Build history of the part. All positions in model axes, mm. A direction names the side the tool comes from. Round coordinates to 2 decimals unless told otherwise and drop trailing zeros. Loops run counter-clockwise (first coordinate to the right, second up) from the corner with the lowest first, then second, coordinate; pieces in that order, holes last.
from build123d import *

# Parameters (mm, degrees)
SKETCH1_W           = 127
SKETCH1_H           = 112.8776
BOSS_EXTRUDE1_DEPTH = 1.778
SKETCH2_R           = 1.27
CUT_EXTRUDE1_DEPTH  = 1.778
BOSS_EXTRUDE2_DEPTH = 9.525
SKETCH4_R           = 1.524
CUT_EXTRUDE2_DEPTH  = 1.0922
LPATTERN1_COUNT     = 2
LPATTERN1_PITCH     = 13.589
BOSS_EXTRUDE3_DEPTH = 9.652
SKETCH6_R           = 1.524
CUT_EXTRUDE3_DEPTH  = 1.016
FILLET1_R           = 1.524
FILLET2_R           = 0.508
LPATTERN2_COUNT     = 2
LPATTERN2_PITCH     = 13.0048
SKETCH7_R           = 1.524
CUT_EXTRUDE4_DEPTH  = 1.016
FILLET3_R           = 0.508
FILLET4_R           = 1.524
SKETCH8_R           = 4.445
BOSS_EXTRUDE4_DEPTH = 8.89


with BuildPart() as part:
    # Sketch1 → Boss-Extrude1 (new body)
    with BuildSketch(Plane(origin=(0, 0, 0), x_dir=(1, 0, 0), z_dir=(0, 1, 0))):
        Rectangle(SKETCH1_W, SKETCH1_H)
    extrude(amount=BOSS_EXTRUDE1_DEPTH)

    # Sketch2 → Cut-Extrude1 (cut)
    with BuildSketch(Plane(origin=(0, 1.778, 0), x_dir=(1, 0, 0), z_dir=(0, 1, 0))):
        with Locations((58.42, 52.1208)):
            Circle(SKETCH2_R)
        with Locations((58.42, -52.1208)):
            Circle(SKETCH2_R)
    extrude(amount=-CUT_EXTRUDE1_DEPTH, mode=Mode.SUBTRACT)

    # Sketch3 → Boss-Extrude2 (add)
    with BuildSketch(Plane(origin=(63.5, 0, 0), x_dir=(0, 0, -1), z_dir=(1, 0, 0))):
        with BuildLine():
            Line((-46.8884, 1.778), (-46.8884, 6.7818))
            ThreePointArc((-46.8884, 6.7818), (-46.739610245, 7.141010245), (-46.3804, 7.2898))
            Line((-46.3804, 7.2898), (-38.4556, 7.2898))
            ThreePointArc((-38.4556, 7.2898), (-38.096389755, 7.141010245), (-37.9476, 6.7818))
            Line((-37.9476, 6.7818), (-37.9476, 1.778))
            Line((-37.9476, 1.778), (-36.8554, 1.778))
            Line((-36.8554, 1.778), (-36.8554, 6.7818))
            ThreePointArc((-36.8554, 6.7818), (-37.324087729, 7.913312271), (-38.4556, 8.382))
            Line((-38.4556, 8.382), (-46.3804, 8.382))
            ThreePointArc((-46.3804, 8.382), (-47.511912271, 7.913312271), (-47.9806, 6.7818))
            Line((-47.9806, 6.7818), (-47.9806, 1.778))
            Line((-47.9806, 1.778), (-46.8884, 1.778))
        make_face()
    boss_extrude2 = extrude(amount=-BOSS_EXTRUDE2_DEPTH)

    # Sketch4 → Cut-Extrude2 (cut)
    with BuildSketch(Plane(origin=(0, 8.382, 0), x_dir=(1, 0, 0), z_dir=(0, 1, 0))):
        with Locations((58.7375, -42.418)):
            Circle(SKETCH4_R)
    cut_extrude2 = extrude(amount=-CUT_EXTRUDE2_DEPTH, mode=Mode.SUBTRACT)

    # LPattern1: Boss-Extrude2, Cut-Extrude2 ×2
    with Locations(*[(0, 0, -i * LPATTERN1_PITCH) for i in range(1, LPATTERN1_COUNT)]):
        add(boss_extrude2)
        add(cut_extrude2, mode=Mode.SUBTRACT)

    # Sketch5 → Boss-Extrude3 (add)
    with BuildSketch(Plane(origin=(60.96, 0, 0), x_dir=(0, 0, -1), z_dir=(1, 0, 0))):
        Polygon((23.4188, 1.778), (23.4188, 8.382), (12.2428, 8.382), (12.2428, 1.778), (13.2588, 1.778), (13.2588, 7.366), (22.4028, 7.366), (22.4028, 1.778), align=None)
    boss_extrude3 = extrude(amount=-BOSS_EXTRUDE3_DEPTH)

    # Sketch6 → Cut-Extrude3 (cut)
    with BuildSketch(Plane(origin=(0, 8.382, 0), x_dir=(1, 0, 0), z_dir=(0, 1, 0))):
        with Locations((56.134, 17.8308)):
            Circle(SKETCH6_R)
    extrude(amount=-CUT_EXTRUDE3_DEPTH, mode=Mode.SUBTRACT)

    # Fillet1
    fillet1_edges = [part.edges().sort_by_distance(p)[0] for p in [
        (56.134, 8.382, -12.2428),
        (56.134, 8.382, -23.4188),
    ]]
    fillet(fillet1_edges, radius=FILLET1_R)

    # Fillet2
    fillet2_edges = [part.edges().sort_by_distance(p)[0] for p in [
        (56.134, 7.366, -22.4028),
        (56.134, 7.366, -13.2588),
    ]]
    fillet(fillet2_edges, radius=FILLET2_R)

    # LPattern2: Boss-Extrude3 ×2
    with Locations(*[(0, 0, i * LPATTERN2_PITCH) for i in range(1, LPATTERN2_COUNT)]):
        add(boss_extrude3)

    # Sketch7 → Cut-Extrude4 (cut)
    with BuildSketch(Plane(origin=(0, 8.382, 0), x_dir=(1, 0, 0), z_dir=(0, 1, 0))):
        with Locations((56.134, 4.826)):
            Circle(SKETCH7_R)
    extrude(amount=-CUT_EXTRUDE4_DEPTH, mode=Mode.SUBTRACT)

    # Fillet3
    fillet3_edges = [part.edges().sort_by_distance(p)[0] for p in [
        (56.134, 7.366, -9.398),
        (56.134, 7.366, -0.254),
    ]]
    fillet(fillet3_edges, radius=FILLET3_R)

    # Fillet4
    fillet4_edges = [part.edges().sort_by_distance(p)[0] for p in [
        (56.134, 8.382, 0.762),
        (56.134, 8.382, -10.414),
    ]]
    fillet(fillet4_edges, radius=FILLET4_R)

    # Sketch8 → Boss-Extrude4 (add)
    with BuildSketch(Plane(origin=(0, 1.778, 0), x_dir=(1, 0, 0), z_dir=(0, 1, 0))):
        with Locations((57.785, -7.1882)):
            Circle(SKETCH8_R)
        with Locations((57.785, -16.8402)):
            Circle(SKETCH8_R)
        with Locations((48.133, -7.1882)):
            Circle(SKETCH8_R)
        with Locations((48.133, -16.8402)):
            Circle(SKETCH8_R)
    extrude(amount=BOSS_EXTRUDE4_DEPTH)


solid = part.part
(1) Slice it at B-B on y = 5. Count the separate pieces of the cut face and the enclosed holes in it, plus the area to 3 significant figures.
Responses:
separate pieces: 12
enclosed holes: 0
area: 329 mm2
(2) Probe line 1 (Y direction, x = -3, z = 25); line 2 (X direction, y = 5.25, z = -10); line 3 (X direction, y = 6, z = 10.5). List the from-to ranges inside material, lowest first.
Responses:
line 1: y = 0 to 1.78
line 2: x = 51.31 to 60.96
line 3: x = 45.17 to 51.1, 54.82 to 60.75
(3) Pin check, flat tips, straight feed: P1, Ø4, axis at x = 3.5, z = 14.5, coming from the +Y side; P2, Ø8.5, axis at x = 56.5, z = 27.5, coming from the +Y side; P3, Ø1.5, axis at x = 54, y = 4, coming from the +Z side; P4, Ø2, axis at y = 3.5, z = -4.5, coming from the +X side. Stop position of each tip, or through.
Responses:
P1: stops at y = 1.78
P2: stops at y = 8.38
P3: stops at z = 47.98
P4: passes through
(4) Slice it at A-A on z = -41.5. List the corners of the cut face in (x, y), plus the area to 3 significant figures.
Responses:
outline: (-63.5, 0) - (63.5, 0) - (63.5, 1.78) - (-63.5, 1.78) - close
area: 226 mm2
(5) Pull direction X, two halves, no side cores. Call faces 1 (the face through (56, 4, -13.259)), 2 (the face through (60.96, 8, -4)), 3 (the face through (43.692, 6.161, 16.645)): +X half, -X half, draft (parallel to the pull), parting line (faces both ways), or undercut.
Responses:
face 1: draft
face 2: +X half
face 3: undercut
(6) Which spindle directions (+Z, -Z, +X, -X, +Y, -Y) get a long thin tool onto all of the face, cutting with end or side? Do faces 4 (the face through (59, 4, 23.266)), 5 (the face through (56, 7.366, -7)), 6 (the face through (43.692, 6.161, 6.993)). Say none if no direction does.
Responses:
face 4: +X, -X, +Y
face 5: +X, -X
face 6: +Y
(7) Slice it at C-C on x = 4. List the corners of the cut face in (y, z), plus the area to 3 significant figures.
Responses:
outline: (0, -56.44) - (1.78, -56.44) - (1.78, 56.44) - (0, 56.44) - close
area: 201 mm2
(8) Slice it at D-D on z = 5.5. List the corners of the cut face in (x, y), plus the area to 3 significant figures.
Responses:
outline: (-63.5, 0) - (63.5, 0) - (63.5, 1.78) - (61.9, 1.78) - (61.9, 10.67) - (53.67, 10.67) - (53.67, 1.78) - (52.24, 1.78) - (52.24, 10.67) - (44.02, 10.67) - (44.02, 1.78) - (-63.5, 1.78) - close
area: 372 mm2
